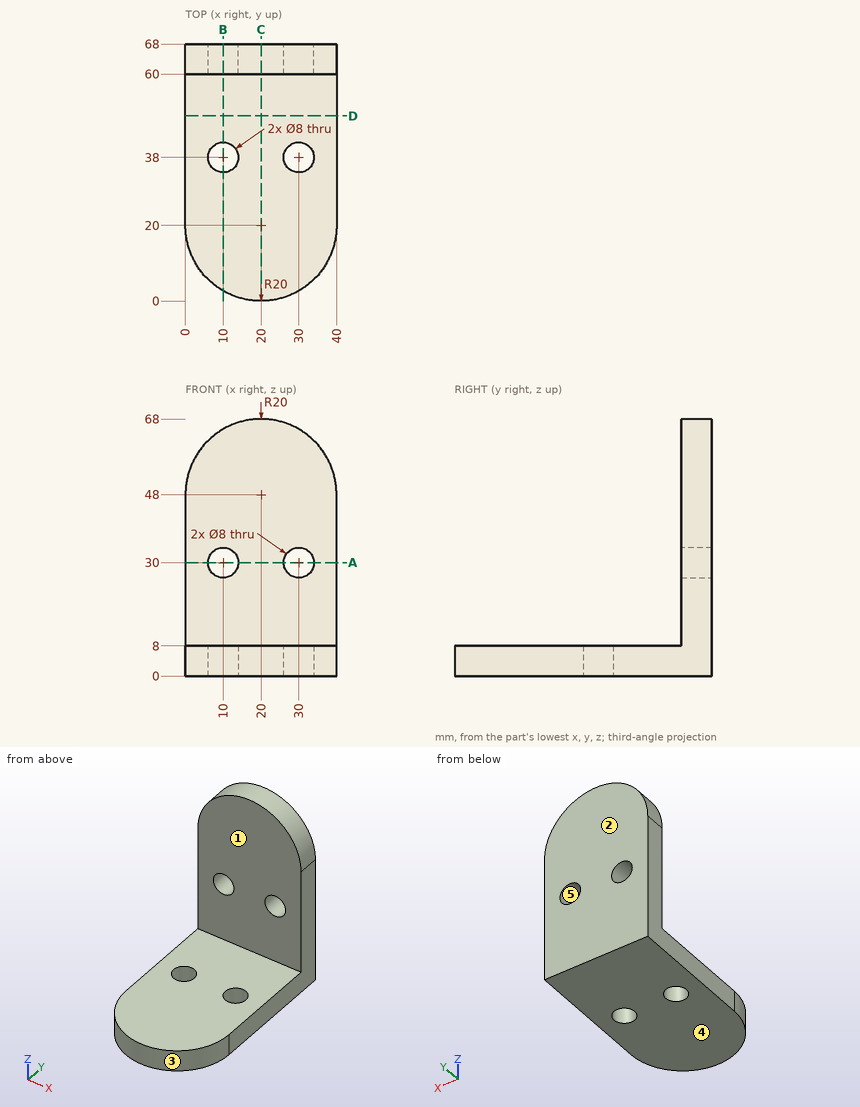
Could you check a few things on this drawing? It's one solid part, dimensions in mm from its lowest x, y, z. A direction names the side the tool comes from. Coordinates: 2 decimals unless noted, no trailing zeros. Order: outer loops, then holes, each group sorted by start corner. A loop starts at its lowest first (then second) coordinate and runs counter-clockwise, first axis right, second up. Notation, with made-up numbers: M 71,37.5 L 104,37.5 A20 cw 104,66.5 Z; hole C 3,79 d4. An arc over 180 degrees is marked long. Use a Markdown table: item, result. Add a question column.
Q1. I want a section at D-D on y = 49. List the corners of the cut face in (x, z) for me.
Q2. I'm going to push flat-ended pins straight in: pin 1 (7 mm diameter, centred on x = 10, y = 38, fed in from +Z); pin 2 (1.5 mm diameter, centred on x = 27, y = 21.5, fed in from +Z); pin 3 (2 mm diameter, centred on x = 24, z = 23, fed in from -Y). Where does each tip first touch, or does it pass through?
Q3. I want a section at B-B on x = 10. List the corners of the cut face in (y, z) for me, then the cut area to 3 significant figures.
Q4. We'd pull the mould along Z, two halves only. Please class the marked faces 3, 4 and 5: pulls with the +Z half, pulls with the -Z half, needs draft (parallel to the pull), parting line crosses it, or undercut.
Q5. I want a section at A-A on z = 30. List the corners of the cut face in (x, y) for me.
Q6. I want a section at C-C on x = 20. List the corners of the cut face in (y, z) for me, then the cut area to 3 significant figures.
Q7. If I drill on L1, parallel to X at y = 64, z = 30; L2, parallel to Z at x = 37, y = 13; L3, parallel to Y at x = 30, z = 44, over which ranges is the centre line in solid material (lowest first)?
Q8. Which directions (+Z, -Z, +X, -X, +Y, -Y) give clear straight access to the entire face, cutting with the end or side of a thin tool? Please do the marked faces 1 and 2.
Checked values:
| question | item | result |
|---|---|---|
| 1 | outline | M 0,0 L 40,0 L 40,8 L 0,8 Z |
| 2 | pin 1 | through |
| 2 | pin 2 | z = 8 |
| 2 | pin 3 | y = 60 |
| 3 | outline | M 2.68,0 L 34,0 L 34,8 L 2.68,8 Z; M 42,0 L 68,0 L 68,26 L 60,26 L 60,8 L 42,8 Z; M 60,34 L 68,34 L 68,65.32 L 60,65.32 Z |
| 3 | area | 853 mm² |
| 4 | face 3 | needs draft |
| 4 | face 4 | pulls with the -Z half |
| 4 | face 5 | undercut |
| 5 | outline | M 0,60 L 6,60 L 6,68 L 0,68 Z; M 14,60 L 26,60 L 26,68 L 14,68 Z; M 34,60 L 40,60 L 40,68 L 34,68 Z |
| 6 | outline | M 0,0 L 68,0 L 68,68 L 60,68 L 60,8 L 0,8 Z |
| 6 | area | 1,020 mm² |
| 7 | L1 | 0 to 6, 14 to 26, 34 to 40 |
| 7 | L2 | 0 to 8 |
| 7 | L3 | 60 to 68 |
| 8 | face 1 | +Z, +X, -X, -Y |
| 8 | face 2 | +Z, -Z, +X, -X, +Y |
